from build123d import *

# Parameters (mm, degrees)
BOSS_EXTRUDE1_DEPTH = 140
BOSS_EXTRUDE2_DEPTH = 36
BOSS_EXTRUDE3_DEPTH = 4
SKETCH3_3_R         = 5
BOSS_EXTRUDE4_DEPTH = 2
SKETCH4_R           = 4.5
CUT_EXTRUDE1_DEPTH  = 184.423008371


with BuildPart() as part:
    # Sketch1 → Boss-Extrude1 (new body)
    with BuildSketch(Plane.XY):
        Polygon((0, 0), (0, 13), (3, 13), (3, 3), (39, 3), (39, 13), (42, 13), (42, 0), align=None)
    extrude(amount=BOSS_EXTRUDE1_DEPTH)

    # Sketch2 → Boss-Extrude2 (add)
    with BuildSketch(Plane.XY.offset(140)):
        Polygon((0, 0), (42, 0), (42, 6), (39, 6), (39, 3), (3, 3), (3, 6), (0, 6), align=None)
    extrude(amount=BOSS_EXTRUDE2_DEPTH)

    # Sketch3 → Boss-Extrude3 (add)
    with BuildSketch(Plane.XY.offset(176)):
        Polygon((0, 17), (0, 6), (3, 6), (3, 3), (39, 3), (39, 6), (42, 6), (42, 17), align=None)
        Polygon((24.75277675, 16.5), (28.505553499, 10), (24.75277675, 3.5), (17.24722325, 3.5), (13.494446501, 10), (17.24722325, 16.5), align=None, mode=Mode.SUBTRACT)
    extrude(amount=-BOSS_EXTRUDE3_DEPTH)

    # Sketch3_3 → Boss-Extrude4 (add)
    # profile 1 of 3: a face of its own
    with BuildSketch(Plane.XY.offset(176)):
        Polygon((3, 6), (0, 6), (0, 0), (42, 0), (42, 6), (39, 6), (39, 3), (3, 3), align=None)
    # profile 2 of 3: a face of its own
    with BuildSketch(Plane.XY.offset(176)):
        Polygon((0, 17), (0, 6), (3, 6), (3, 3), (39, 3), (39, 6), (42, 6), (42, 17), align=None)
        Polygon((24.75277675, 16.5), (28.505553499, 10), (24.75277675, 3.5), (17.24722325, 3.5), (13.494446501, 10), (17.24722325, 16.5), align=None, mode=Mode.SUBTRACT)
    # profile 3 of 3: a face of its own
    with BuildSketch(Plane.XY.offset(176)):
        Polygon((17.24722325, 3.5), (24.75277675, 3.5), (28.505553499, 10), (24.75277675, 16.5), (17.24722325, 16.5), (13.494446501, 10), align=None)
        with Locations((21, 10)):
            Circle(SKETCH3_3_R, mode=Mode.SUBTRACT)
    extrude(amount=BOSS_EXTRUDE4_DEPTH)

    # Sketch4 → Cut-Extrude1 (cut, through all)
    with BuildSketch(Plane(origin=(0, 3, 0), x_dir=(1, 0, 0), z_dir=(0, 1, 0))):
        with Locations(Location((21, -152, 0), (0, 0, 270))):
            Circle(SKETCH4_R)
        with Locations(Location((21, -71.075, 0), (0, 0, 270))):
            Circle(SKETCH4_R)
    extrude(amount=-CUT_EXTRUDE1_DEPTH, mode=Mode.SUBTRACT)


solid = part.part
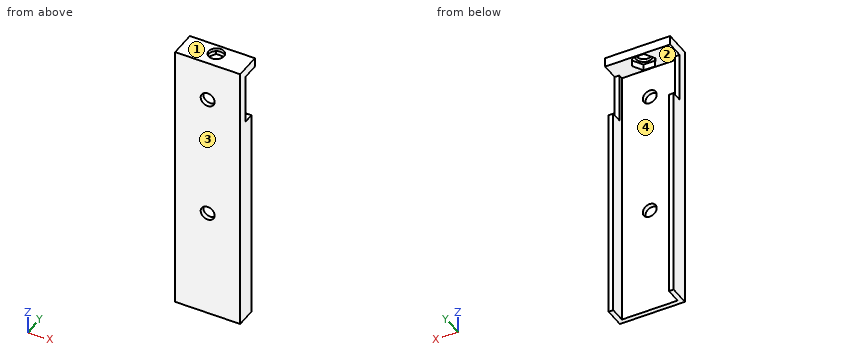
For this review, take the finished solid that the model builds, in its own axes (mm). Face numbers are marked on the shaded views. A direction names the side the tool comes from. Give positions to 0.01 mm unless a question says otherwise; leave off trailing zeros. Loops run counter-clockwise (first coordinate to the right, second up) from the corner with the lowest first, then second, coordinate; pieces in that order, holes last. Notation, with made-up numbers: M 11,60.5 L 69,60.5 A17 ccw 69,79.5 Z; hole C 46.25,44 d1. An arc over 180 degrees is marked long. Answer as a JSON object with one key per item and string values. Group by question number.
Q1. Add section A-A on x = 21. Give the boundary of the cut face in (y, z) (3 decimals).
Q2. Add section C-C on y = 8.5. Give the boundary of the cut face in (x, z), and give its area (3 significant figures).
Q3. Insertion check: P1, Ø7, axis at x = 15.5, y = 10.5, coming from the -Z side; P2, Ø1.5, axis at x = 33, z = 36.5, coming from the +Y side; P3, Ø0.9, axis at x = 41, z = 155.5, coming from the +Y side; P4, Ø8, axis at y = 6.5, z = 64.5, coming from the -X side. Each pin has a flat end and moves straight along its axis. Give the tip position at first contact, or say it passes through.
Q4. Add section B-B on z = 152. Give the boundary of the cut face in (x, y), and give its area (3 significant figures).
Q5. For probe 1 along X at (y, z) = (5.75, 44.5); probe 2 along Y at (x, z) = (11.5, 156); probe 3 along Y at (x, z) = (21, 177.1), list the stretches that pass through material, from the lowest coordinate up. Write a range as [from, to].
Q6. Mouldability with a two-part tool opening along X and no side actions: class the marked faces 3 and 4 as +X half, -X half, draft (parallel to the pull), parting line (faces both ways), or undercut.
Q7. Add section D-D on x = 4.5. Give the boundary of the cut face in (y, z).
Q8. Tool access review of the marked faces 1 and 2: name each direction out of +Z, -Z, +X, -X, +Y, -Y from which nothing blocks a thin tool from reaching the whole face with its end or side.
Checked values:
{
 "1": {"outline": "M 0,0 L 3,0 L 3,66.575 L 0,66.575 Z; M 0,75.575 L 3,75.575 L 3,147.5 L 0,147.5 Z; M 0,156.5 L 3,156.5 L 3,172 L 3.5,172 L 3.5,176 L 5,176 L 5,178 L 0,178 Z; M 15,176 L 16.5,176 L 16.5,172 L 17,172 L 17,178 L 15,178 Z"},
 "2": {"outline": "M 0,0 L 3,0 L 3,140 L 0,140 Z; M 0,172 L 14.36,172 L 14.36,176 L 16.23,176 L 16.23,178 L 0,178 Z; M 25.77,176 L 27.64,176 L 27.64,172 L 42,172 L 42,178 L 25.77,178 Z; M 39,0 L 42,0 L 42,140 L 39,140 Z", "area": "1,020 mm²"},
 "3": {"P1": "z = 172", "P2": "y = 3", "P3": "y = 6", "P4": "x = 0"},
 "4": {"outline": "M 0,0 L 16.5,0 L 16.5,3 L 3,3 L 3,6 L 0,6 Z; M 25.5,0 L 42,0 L 42,6 L 39,6 L 39,3 L 25.5,3 Z", "area": "117 mm²"},
 "5": {"probe 1": "[0, 3], [39, 42]", "probe 2": "[0, 3]", "probe 3": "[0, 5], [15, 17]"},
 "6": {"face 3": "draft", "face 4": "undercut"},
 "7": {"outline": "M 0,0 L 3,0 L 3,172 L 17,172 L 17,178 L 0,178 Z"},
 "8": {"face 1": "+Z, +X, -X, +Y, -Y", "face 2": "+Y"}
}
